Can you work these out from the model? Positions are in its coordinate system, mm. A direction names the side the tool comes from. Round coordinates to 2 decimals unless told otherwise and drop trailing zeros. Write each loop counter-clockwise with the first axis right and the second up, starting at its lowest first coordinate (ties: lowest second). Pieces come first, ordered by that corner, then holes. Notation, with made-up numbers: (86, 43.5) - (103, 43.5) arc R6 ccw to (103, 47.5) - close; hole circle Ø5 at (0.25, -8). An arc over 180 degrees is marked (long way). One line per item, written item: value. Start each with the question number.
(1) I want a section at A-A on z = 93. List the corners of the cut face in (x, y) for me.
(2) I'm going to push flat-ended pins straight in: pin 1 Ø1.5 at (y, z) = (14, 15) entering from +X; pin 2 Ø3 at (x, y) = (17, 13) entering from -Z; pin 3 Ø1 at (y, z) = (12.5, 35) entering from -X. Where does each tip first touch, or does it pass through?
(3) On a 3-axis mill with a long thin cutter (end or side, diameter ignored), from which of +Z, -Z, +X, -X, +Y, -Y can I reach the whole of each face in a straight line? I mean faces 1 (the face through (15.6, 11.37, 75.13)), 2 (the face through (18.5, 9.5, 152.4)), 3 (the face through (21.53, 14.816, 63.05)), 4 (the face through (21.54, 11.39, 75.13)). Say none if no direction works.
(4) If I drill on L1, parallel to Y at x = 20, z = 8; L2, parallel to X at y = 12.75, z = 155; L3, parallel to Y at x = 19.5, z = 162.5, over which ranges is the centre line in solid material (lowest first)? Write a range as from..to.
from build123d import *

# Parameters (mm, degrees)
F1_DEPTH = 152.4
F3_DEPTH = 12.7
F4_R     = 3.7116770234
F5_DEPTH = 6.35
F7_R     = 0.2026181046


with BuildPart() as f1:
    # F0 (on Top) → F1 (new body)
    with BuildSketch(Plane.XY):
        Polygon((22.5227356887, 13.1351892635), (20.5084380472, 16.5440003483), (16.5491722304, 16.5039729623), (14.604204055, 13.0551344916), (16.6185016965, 9.6463234069), (20.5777675134, 9.6863507928), align=None)
    extrude(amount=F1_DEPTH)

    # F1_face (on face) + F1_face1 (on face) + F2 (on face) → F3 (join)
    with BuildSketch(Plane(origin=(18.5634698719, 13.0951618776, 152.4), x_dir=(1, 0, 0), z_dir=(0, 0, 1))):
        Polygon((3.9592658168, 0.0400273859), (1.9449681753, 3.4488384707), (-2.0142976415, 3.4088110847), (-3.9592658168, -0.0400273859), (-1.9449681753, -3.4488384707), (2.0142976415, -3.4088110847), align=None)
    with BuildSketch(Plane(origin=(18.5634698719, 13.0951618776, 0), x_dir=(1, 0, 0), z_dir=(0, 0, -1))):
        Polygon((1.9449681753, -3.4488384707), (3.9592658168, -0.0400273859), (2.0142976415, 3.4088110847), (-1.9449681753, 3.4488384707), (-3.9592658168, 0.0400273859), (-2.0142976415, -3.4088110847), align=None)
    with BuildSketch(Plane.XY.offset(152.4)):
        with BuildLine():
            ThreePointArc((14.604204055, 13.0551344916), (18.5753456023, 9.1190642761), (22.5231408121, 13.0785499639))
            ThreePointArc((22.5231408121, 13.0785499639), (22.5230395299, 13.1068703381), (22.5227356887, 13.1351892635))
            Line((22.5227356887, 13.1351892635), (20.5777675134, 9.6863507928))
            Line((20.5777675134, 9.6863507928), (16.6185016965, 9.6463234069))
            Line((16.6185016965, 9.6463234069), (14.604204055, 13.0551344916))
        make_face()
        with BuildLine():
            Line((20.5230763012, 16.5192279208), (22.5227356887, 13.1351892635))
            ThreePointArc((22.5227356887, 13.1351892635), (21.9724789039, 15.0928653351), (20.5230763012, 16.5192279208))
        make_face()
        with BuildLine():
            Line((20.5777675134, 9.6863507928), (22.5227356887, 13.1351892635))
            Line((22.5227356887, 13.1351892635), (20.5230763012, 16.5192279208))
            ThreePointArc((20.5230763012, 16.5192279208), (20.501303397, 16.5315365084), (20.4794531772, 16.543707317))
            Line((20.4794531772, 16.543707317), (16.5781571004, 16.5042659936))
            ThreePointArc((16.5781571004, 16.5042659936), (16.5565574105, 16.491655915), (16.5350378058, 16.4789096488))
            Line((16.5350378058, 16.4789096488), (14.604204055, 13.0551344916))
            Line((14.604204055, 13.0551344916), (16.6185016965, 9.6463234069))
            Line((16.6185016965, 9.6463234069), (20.5777675134, 9.6863507928))
        make_face()
        with BuildLine():
            ThreePointArc((16.5350378058, 16.4789096488), (15.1147689879, 15.0235352587), (14.604204055, 13.0551344916))
            Line((14.604204055, 13.0551344916), (16.5350378058, 16.4789096488))
        make_face()
        with BuildLine():
            Line((16.5781571004, 16.5042659936), (20.4794531772, 16.543707317))
            ThreePointArc((20.4794531772, 16.543707317), (18.5236100767, 17.0378506299), (16.5781571004, 16.5042659936))
        make_face()
    extrude(amount=F3_DEPTH, dir=(0, 0, 1))

    # F4 (on face) → F5 (join)
    with BuildSketch(Plane.XY.offset(165.1)):
        with Locations((18.563637815, 13.0785499639)):
            Circle(F4_R)
    extrude(amount=F5_DEPTH)

    # F1_face1 (on face) → F8 section 0
    with BuildSketch(Plane(origin=(18.5634698719, 13.0951618776, 0), x_dir=(1, 0, 0), z_dir=(0, 0, -1))):
        Polygon((1.9449681753, -3.4488384707), (3.9592658168, -0.0400273859), (2.0142976415, 3.4088110847), (-1.9449681753, 3.4488384707), (-3.9592658168, 0.0400273859), (-2.0142976415, -3.4088110847), align=None)
    # F7 (on offset) → F8 section 1
    with BuildSketch(Plane(origin=(0, 0, -12.7), x_dir=(1, 0, 0), z_dir=(0, 0, -1))):
        with Locations((18.5634698719, -13.0951618776)):
            Circle(F7_R)
    loft()


solid = f1.part
Established:
1. outline: (14.6, 13.06) - (16.62, 9.65) - (20.58, 9.69) - (22.52, 13.14) - (20.51, 16.54) - (16.55, 16.5) - close
2. pin 1: x = 22.45
2. pin 2: z = -12.7
2. pin 3: x = 14.64
3. face 1: -Z, -X, -Y
3. face 2: -Z, -Y
3. face 3: -Z, +X, +Y
3. face 4: -Z, +X, -Y
4. L1: 9.68..16.54
4. L2: 14.62..22.51
4. L3: 9.23..16.93
